Geometry: final body of the model. Coordinates: model frame, mm. A direction names the side the tool comes from. Round coordinates to 2 decimals unless told otherwise and drop trailing zeros. Loops run counter-clockwise (first coordinate to the right, second up) from the corner with the lowest first, then second, coordinate; pieces in that order, holes last. Notation, with made-up numbers: (-38, 32) -> (-4, 32) arc R15 ccw to (-4, 37) -> close; hole circle Ø2 at (52.25, 83). An arc over 180 degrees is marked (long way). Answer in a Markdown table with one row per item.
Autodesk Inventor part; units mm, degrees
ref_plane "YZ Plane" through (0, 0, 0) normal (1, 0, 0) x (0, 1, 0)
ref_plane "XZ Plane" through (0, 0, 0) normal (0, 1, 0) x (-1, 0, 0)
ref_plane "XY Plane" through (0, 0, 0) normal (0, 0, 1) x (1, 0, 0)
sketch "Sketch1" plane through (0, 0, 0) normal (0, 1, 0) x (-1, 0, 0)
  line L0 (0, 0) -> (30, 0)
  line L1 (30, 0) -> (30, -65)
  line L2 (30, -65) -> (0, -65)
  line L3 (0, -65) -> (0, 0)
  line L4 (-20, 10) -> (36.5, 10)
  line L5 (36.5, 10) -> (36.5, -75)
  line L6 (36.5, -75) -> (-20, -75)
  line L7 (-20, -75) -> (-20, 10)
  circle A0 centre (30, 0) radius 1.5
  circle A1 centre (30, -65) radius 1.5
  circle A2 centre (0, 0) radius 1.5
  circle A3 centre (0, -65) radius 1.5
  dimension "d0" = 30
  dimension "d1" = 65
  dimension "d2" = 10
  dimension "d3" = 6.5
  dimension "d4" = 10
  dimension "d5" = 20
  dimension "d6" = 3
  dimension "d7" = 3
  dimension "d8" = 3
  dimension "d9" = 3
extrude "Extrusion1" add sketch "Sketch1" along normal blind 15 contours L0 A0 L1 A1 L2 A3 L3 A2 | L4 L5 L6 L7
sketch "Sketch2" plane through (20, 0, 10) normal (1, 0, 0) x (0, 0, -1)
  line L0 (0, 0) -> (0, 15)
  line L1 (85, 0) -> (85, 15)
  line L2 (42.5, 4.7) -> (42.5, 11.9085)
  circle A0 centre (17.5, 4.7) radius 2.675
  circle A1 centre (67.5, 4.7) radius 2.675
  line L3 (0, 4.7) -> (85, 4.7)
  line L4 (0, 0) -> (85, 0)
  line L5 (0, 10.3) -> (85, 10.3)
  circle A2 centre (25, 10.3) radius 2.675
  circle A3 centre (60, 10.3) radius 2.675
  line L6 (0, 15) -> (85, 15)
  line L7 (17.5, 7.375) -> (26.8128, 7.375)
  point P0 (10, 0)
  dimension "d12" = 5.35
  dimension "d13" = 5.35
  dimension "d26" = 4.7
  dimension "d27" = 5.35
  dimension "d28" = 5.35
  dimension "d29" = 4.7
  dimension "d31" = 17.5
  dimension "d32" = 17.5
  dimension "d33" = 25
  dimension "d34" = 25
extrude "Extrusion2" cut sketch "Sketch2" against normal blind 43 contours L3 A0 | A0 L3 | A2 L5 | L5 A2 | L3 A1 | A1 L3 | A3 L5 | L5 A3
sketch "Sketch3" plane through (0, 15, 0) normal (0, 1, 0) x (1, 0, 0)
  circle A0 centre (-30, 0) radius 1.5
  circle A1 centre (-30, 0) radius 4
  circle A2 centre (-30, 65) radius 1.5
  circle A3 centre (-30, 65) radius 4
  circle A4 centre (0, 0) radius 1.5
  circle A5 centre (0, 0) radius 4
  circle A6 centre (0, 65) radius 1.5
  circle A7 centre (0, 65) radius 4
  dimension "d18" = 8
  dimension "d19" = 8
  dimension "d20" = 8
  dimension "d21" = 8
extrude "Extrusion3" cut sketch "Sketch3" against normal blind 7.5 contours A0 | A1 | A3 | A5 | A7
fillet "Fillet1" radius 15 4 edges at (-36.5, 7.5, 10) (20, 7.5, 10) (20, 7.5, -75) (-36.5, 7.5, -75)
sketch "Sketch4" plane through (-36.5, 0, -60) normal (-1, 0, 0) x (0, 0, 1)
  point P0 (60, 0)
fillet "Fillet3" radius 3 8 edges at (15.6066, 15, -70.6066) (-8.25, 15, -75) (-32.1066, 15, -70.6066) (-36.5, 15, -32.5) (-32.1066, 15, 5.6066) (-8.25, 15, 10) (15.6066, 15, 5.6066) (20, 15, -32.5)
properties part number "BaseStabilizerAttachment"
Item 1: Draft query along Y for faces 4 (the face through (0, 7.5, -63)), 5 (the face through (-23, 5, -7)), 6 (the face through (-36.5, 6, -32)). Return one class per face: pulls with the +Y half, pulls with the -Y half, needs draft (parallel to the pull), parting line crosses it, or undercut.
Answer:
| item | result |
|---|---|
| face 4 | pulls with the +Y half |
| face 5 | undercut |
| face 6 | needs draft |
Item 2: Line query: probe 1 along Z at (x, y) = (-12, 10); probe 2 along Z at (x, y) = (0, 10); probe 3 along Z at (x, y) = (3.5, 5.25). Output: solid intervals per line, ascending. Write a range as [from, to].
Answer:
| item | result |
|---|---|
| probe 1 | z = [-75, -52.66], [-47.34, -17.66], [-12.34, 10] |
| probe 2 | z = [-75, -69], [-61, -52.66], [-47.34, -17.66], [-12.34, -4], [4, 10] |
| probe 3 | z = [-75, -60.12], [-54.88, -10.12], [-4.88, 10] |
Item 3: Reachability of faces 1 (the face through (-1.2, 3.07, -5.38)), 2 (the face through (-8.06, 14.14, 9.1)), 3 (the face through (-28, 7.5, 0)) from +Z, -Z, +X, -X, +Y, -Y: full face, straight path, thin tool, end or side. Return the list, or none.
Answer:
| item | result |
|---|---|
| face 1 | +X |
| face 2 | +Z, +X, -X, +Y |
| face 3 | +Y |
Item 4: Cut plane C-C (z = -50). Output: boundary loops of the cut face in (x, y) (3 decimals).
Answer:
| item | result |
|---|---|
| outline | (-36.5, 0) -> (20, 0) -> (20, 7.625) -> (-23, 7.625) -> (-23, 12.975) -> (19.837, 12.975) arc R3 ccw to (17, 15) -> (-33.5, 15) arc R3 ccw to (-36.5, 12) -> close |
Item 5: Cut plane A-A (x = -5). Output: boundary loops of the cut face in (y, z) (3 decimals), then the cut area to 3 significant figures.
Answer:
| item | result |
|---|---|
| outline | (0, -75) -> (12, -75) arc R3 ccw to (15, -72) -> (15, 7) arc R3 ccw to (12, 10) -> (0, 10) -> close; hole circle Ø5.35 at (4.7, -57.5); hole circle Ø5.35 at (4.7, -7.5); hole circle Ø5.35 at (10.3, -50); hole circle Ø5.35 at (10.3, -15) |
| area | 1,180 mm² |
Item 6: Cut plane B-B (z = -7.5). Output: boundary loops of the cut face in (x, y) (3 decimals), then the cut area to 3 significant figures.
Answer:
| item | result |
|---|---|
| outline | (-36.5, 0) -> (20, 0) -> (20, 2.025) -> (-23, 2.025) -> (-23, 7.375) -> (20, 7.375) -> (20, 12) arc R3 ccw to (17, 15) -> (-33.5, 15) arc R3 ccw to (-36.5, 12) -> close |
| area | 614 mm² |
Item 7: Pin query (flat end, axial travel): pin 1 Ø1.5 at (y, z) = (4, -2) entering from +X; pin 2 Ø3.5 at (x, z) = (0, 0) entering from +Y; pin 3 Ø2 at (y, z) = (8.5, 1) entering from +X. Return the tip coordinate at first contact, or that it passes through.
Answer:
| item | result |
|---|---|
| pin 1 | stops at x = 19.83 |
| pin 2 | stops at y = 7.5 |
| pin 3 | stops at x = 19.14 |
